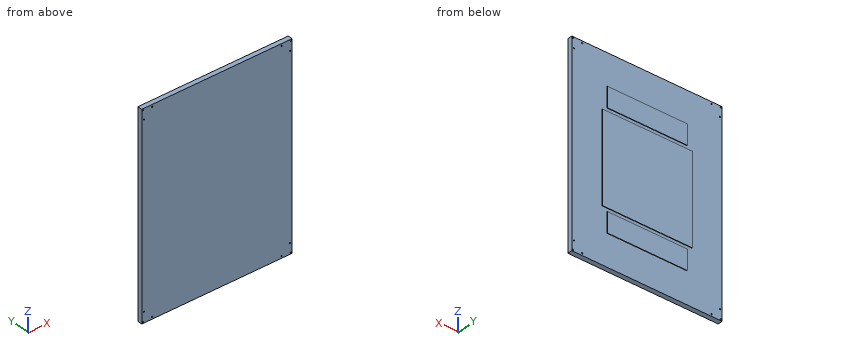
Autodesk Inventor part; units mm, degrees
ref_plane "YZ Plane" through (0, 0, 0) normal (1, 0, 0) x (0, 1, 0)
ref_plane "XZ Plane" through (0, 0, 0) normal (0, 1, 0) x (-1, 0, 0)
ref_plane "XY Plane" through (0, 0, 0) normal (0, 0, 1) x (1, 0, 0)
sketch "Эскиз1" plane through (0, 0, 0) normal (0, 1, 0) x (-1, 0, 0)
  line L0 (-225, 300) -> (225, 300)
  line L1 (225, 300) -> (225, -300)
  line L2 (225, -300) -> (-225, -300)
  line L3 (-225, -300) -> (-225, 300)
  line L4 (-225, 300) -> (225, -300) construction
  line L5 (225, 300) -> (-225, -300) construction
  line L6 (-135, 135) -> (135, 135)
  line L7 (135, 135) -> (135, -135)
  line L8 (135, -135) -> (-135, -135)
  line L9 (-135, -135) -> (-135, 135)
  line L10 (-135, 135) -> (135, -135) construction
  line L11 (135, 135) -> (-135, -135) construction
  line L12 (120, 145) -> (-120, 145)
  line L13 (-120, 145) -> (-120, 205)
  line L14 (-120, 205) -> (120, 205)
  line L15 (120, 205) -> (120, 145)
  line L16 (120, -145) -> (-120, -145)
  line L17 (-120, -145) -> (-120, -205)
  line L18 (-120, -205) -> (120, -205)
  line L19 (120, -205) -> (120, -145)
  point P0 (0, 0)
  dimension "d0" = 450
  dimension "d1" = 600
  dimension "d2" = 270
  dimension "d3" = 270
  dimension "d7" = 240
  dimension "d8" = 60
  dimension "d9" = 60
  dimension "d10" = 15
  dimension "d11" = 10
  dimension "d12" = 10
  dimension "d13" = 15
extrude "Выдавливание1" add sketch "Эскиз1" along normal blind 14
extrude "Выдавливание2" add sketch "Эскиз1" along normal blind 15.5 contours L6 L7 L8 L9 | L12 L13 L14 L15 | L19 L18 L17 L16
sketch "Эскиз2" plane through (0, 14, 0) normal (0, 1, 0) x (1, 0, 0)
  circle A0 centre (-193.75, 293.75) radius 1.75
  circle A1 centre (-218.75, 268.75) radius 1.75
  circle A2 centre (-221, 296) radius 1.75
  circle A3 centre (221, 296) radius 1.75
  circle A4 centre (218.75, 268.75) radius 1.75
  circle A5 centre (193.75, 293.75) radius 1.75
  circle A6 centre (218.75, -268.75) radius 1.75
  circle A7 centre (221, -296) radius 1.75
  circle A8 centre (193.75, -293.75) radius 1.75
  circle A9 centre (-218.75, -268.75) radius 1.75
  circle A10 centre (-221, -296) radius 1.75
  circle A11 centre (-193.75, -293.75) radius 1.75
  line L0 (225, 300) -> (-225, 300)
  line L1 (-225, 300) -> (-225, -300)
  line L2 (225, -300) -> (225, 300)
  line L3 (-225, -300) -> (225, -300)
  point P0 (0, 0)
  dimension "d20" = 27.25
  dimension "d21" = 27.25
  dimension "d22" = 2.25
  dimension "d23" = 2.25
  dimension "d24" = 4
  dimension "d25" = 4
  dimension "d26" = 27.25
  dimension "d27" = 27.25
  dimension "d28" = 2.25
  dimension "d29" = 2.25
  dimension "d30" = 4
  dimension "d31" = 4
  dimension "d32" = 27.25
  dimension "d33" = 27.25
  dimension "d34" = 2.25
  dimension "d35" = 2.25
  dimension "d36" = 4
  dimension "d37" = 4
  dimension "d38" = 27.25
  dimension "d39" = 27.25
  dimension "d40" = 2.25
  dimension "d41" = 2.25
  dimension "d42" = 4
  dimension "d43" = 4
extrude "Выдавливание3" cut sketch "Эскиз2" against normal through all contours A0 | A1 | A2 | A3 | A4 | A5 | A6 | A7 | A8 | A9 | A10 | A11
properties part number "base_plate"
The listing builds one solid part. Answer for the finished solid, in the listing's coordinates (mm). Round coordinates to 2 decimals unless told otherwise and drop trailing zeros. Loops run counter-clockwise (first coordinate to the right, second up) from the corner with the lowest first, then second, coordinate; pieces in that order, holes last. Notation, with made-up numbers: (70, -29.75) - (77, -29.75) arc R34 ccw to (77, 7.25) - close; hole circle Ø4 at (81, 80). An arc over 180 degrees is marked (long way). Return JSON: item names as keys, results as strings. Group by question number.
1. Each of these flat-tipped pins is pushed along its axis until it touches: P1, Ø4, axis at x = -221, z = 296, coming from the +Y side; P2, Ø1.2, axis at x = -23.5, y = 15, coming from the +Z side; P3, Ø1.2, axis at y = 15, z = 170.5, coming from the +X side. Where does it stop, or does it pass through?
2. The part is cut by section D-D on x = -171.5. Determine the outline of the cut face in (y, z).
3. The part is cut by section B-B on z = -3.5. Determine the outline of the cut face in (x, y).
4. The part is cut by section A-A on x = -2.5. Determine the outline of the cut face in (y, z).
5. Consider probe 1 along X at (y, z) = (4, -293.75); probe 2 along X at (y, z) = (6.5, -296); probe 3 along Z at (x, y) = (-221, 8.5). Determine where each line is inside the solid, lowest interval first.
6. The part is cut by section C-C on z = 182.5. Determine the outline of the cut face in (x, y), then the cut area to 3 significant figures.
Resolved:
{
 "1": {"P1": "stops at y = 14", "P2": "stops at z = 205", "P3": "stops at x = 120"},
 "2": {"outline": "(0, -300) - (14, -300) - (14, 300) - (0, 300) - close"},
 "3": {"outline": "(-225, 0) - (225, 0) - (225, 14) - (135, 14) - (135, 15.5) - (-135, 15.5) - (-135, 14) - (-225, 14) - close"},
 "4": {"outline": "(0, -300) - (14, -300) - (14, -205) - (15.5, -205) - (15.5, -145) - (14, -145) - (14, -135) - (15.5, -135) - (15.5, 135) - (14, 135) - (14, 145) - (15.5, 145) - (15.5, 205) - (14, 205) - (14, 300) - (0, 300) - close"},
 "5": {"probe 1": "x = -225 to -195.5, -192 to 192, 195.5 to 225", "probe 2": "x = -225 to -222.75, -219.25 to 219.25, 222.75 to 225", "probe 3": "z = -300 to -297.75, -294.25 to 294.25, 297.75 to 300"},
 "6": {"outline": "(-225, 0) - (225, 0) - (225, 14) - (120, 14) - (120, 15.5) - (-120, 15.5) - (-120, 14) - (-225, 14) - close", "area": "6,660 mm²"}
}
